Read the model definition and answer for the solid it produces. Units are mm, in the model's axes. A direction names the side the tool comes from. Coordinates: 2 decimals unless noted, no trailing zeros. Order: outer loops, then holes, each group sorted by start corner. A loop starts at its lowest first (then second) coordinate and runs counter-clockwise, first axis right, second up. Notation, with made-up numbers: (14, -13) -> (65, -13) arc R21 ccw to (65, 12) -> close; hole circle Ø4 at (-9.5, 5). An arc over 180 degrees is marked (long way). Use CSV: the item, a comma, the result in double quotes.
```python
from build123d import *

# Parameters (mm, degrees)
SM_BASE_FLANGE_1_DEPTH = 975


# Sheet-metal steps are written as plain solids
with BuildPart() as part:
    # Sketch 1 → Базовая кромка1 (new body)
    with BuildSketch(Plane(origin=(0, 0, 0), x_dir=(1, 0, 0), z_dir=(0, 1, 0))):
        with BuildLine():
            Line((0, 0), (29.799038106, 0))
            ThreePointArc((29.799038106, 0), (29.99315239, 0.02555563), (30.174038106, 0.100480947))
            Line((30.174038106, 0.100480947), (69.199028853, 22.63156986))
            ThreePointArc((69.199028853, 22.63156986), (69.862276479, 22.906296022), (70.574028853, 23))
            Line((70.574028853, 23), (99.837168574, 23))
            Line((99.837168574, 23), (99.837168574, 21))
            Line((99.837168574, 21), (70.574028853, 21))
            ThreePointArc((70.574028853, 21), (70.379914569, 20.97444437), (70.199028853, 20.899519053))
            Line((70.199028853, 20.899519053), (31.174038106, -1.63156986))
            ThreePointArc((31.174038106, -1.63156986), (30.51079048, -1.906296022), (29.799038106, -2))
            Line((29.799038106, -2), (0, -2))
            Line((0, -2), (0, 0))
        make_face()
    extrude(amount=SM_BASE_FLANGE_1_DEPTH)

    # Зеркальное отражение1: part across plane


with BuildPart() as part_1:
    add(part.part)
    add(part.part.mirror(Plane(origin=(0, 1077.919678531, 2), x_dir=(0, 0, 1), z_dir=(-1, 0, 0))))

    # Зеркальное отражение2: part across plane


with BuildPart() as part_2:
    add(part_1.part)
    add(part_1.part.mirror(Plane(origin=(31, 975, 1.732050808), x_dir=(0, 0, 1), z_dir=(0, 1, 0))))


solid = part_2.part
```
Item 1: Each of these flat-tipped pins is pushed along its axis until it touches: P1, Ø14.5, axis at x = -91, y = 1177.5, coming from the +Z side; P2, Ø1, axis at x = -68, z = -19, coming from the -Y side; P3, Ø2, axis at y = 420, z = -11.5, coming from the +X side; P4, Ø10, axis at x = 63.5, y = 466, coming from the +Z side. Where does it stop, or does it pass through?
Return value:
P1,"stops at z = -21"
P2,"passes through"
P3,"stops at x = 55.65"
P4,"stops at z = -14.15"
Item 2: The mould has two halves that part along X. Classify faces 3 (the flat face through (0, 989, 0)), 4 (the flat face through (-50.96, 988.65, -9.79)), 5 (the flat face through (50.96, 988.65, -9.79)): +X half, -X half, draft (parallel to the pull), parting line (faces both ways), or undercut.
Return value:
face 3,"undercut"
face 4,"-X half"
face 5,"+X half"
Item 3: Find section C-C, the plane x = -13. Give the vertices of the cut face in (y, z).
Return value:
outline,"(0, 0) -> (1950, 0) -> (1950, 2) -> (0, 2) -> close"
Item 4: Straight lines are drawn through the part: line 1 along Z through (x, y) = (-2, 1233.5); line 2 along X through (y, z) = (601.5, -1.5); line 3 along X through (y, z) = (522, -19). For each, find the intervals that lie inside material, in ascending order.
Return value:
line 1,"z = 0 to 2"
line 2,"x = -36.6 to -32.6, 32.6 to 36.6"
line 3,"x = -66.91 to -62.91, 62.91 to 66.91"
Item 5: Find section B-B, the plane y = 1139.5. Give the vertices of the cut face in (x, z).
Return value:
outline,"(-99.84, -23) -> (-70.57, -23) arc R2.75 ccw to (-69.2, -22.63) -> (-30.17, -0.1) arc R0.75 cw to (-29.8, 0) -> (29.8, 0) arc R0.75 cw to (30.17, -0.1) -> (69.2, -22.63) arc R2.75 ccw to (70.57, -23) -> (99.84, -23) -> (99.84, -21) -> (70.57, -21) arc R0.75 cw to (70.2, -20.9) -> (31.17, 1.63) arc R2.75 ccw to (29.8, 2) -> (-29.8, 2) arc R2.75 ccw to (-31.17, 1.63) -> (-70.2, -20.9) arc R0.75 cw to (-70.57, -21) -> (-99.84, -21) -> close"
Item 6: Find section A-A, the plane z = -11. Give the vertices of the cut face in (x, y).
Return value:
outline,"(-53.05, 0) -> (-49.05, 0) -> (-49.05, 1950) -> (-53.05, 1950) -> close; (49.05, 0) -> (53.05, 0) -> (53.05, 1950) -> (49.05, 1950) -> close"
Item 7: A tool of negligible diameter and unlimited length cuts with its end or side. For faces 1 (the flat face through (0, 989, 2)), 2 (the flat face through (-49.4, 988.6, -11.2)), from which of +Z, -Z, +X, -X, +Y, -Y can it reach the whole face along a straight path? Write none if from no direction.
Return value:
face 1,"+Z, +X, -X, +Y, -Y"
face 2,"-Z, +Y, -Y"
